Source: CAD feature listing. Evaluate the final solid. Frame: model axes, mm. A direction names the side the tool comes from. Coordinates: 2 decimals unless noted, no trailing zeros. Loops run counter-clockwise (first coordinate to the right, second up) from the corner with the lowest first, then second, coordinate; pieces in that order, holes last.
Item 1: Section query C-C, the plane y = 13. Return the cut outline in (x, z), then the cut area to 3 significant figures.
Item 2: Section query A-A, the plane x = 18. Return the cut outline in (y, z), then the cut area to 3 significant figures.
Item 3: Reachability of faces 1 (the flat face through (0, -26, 0)), 2 (the flat face through (-10.465, -7.697, 76.75)), 3 (the flat face through (-0.09, -47.92, 117.41)), 4 (the cylindrical face through (10.54, -18.81, 69)) from +Z, -Z, +X, -X, +Y, -Y: full face, straight path, thin tool, end or side. Return the list, or none.
Item 4: Pin query (flat end, axial travel): pin 1 Ø5 at (y, z) = (17, -5) entering from -X; pin 2 Ø10 at (x, y) = (-2.5, -21.5) entering from +Z; pin 3 Ø1.5 at (y, z) = (-12.5, 46.5) entering from -X; pin 4 Ø5 at (x, y) = (5.5, -40) entering from -Z. Return the tip coordinate at first contact, or that it passes through.
Item 5: Section query D-D, the plane x = -2. Return the cut outline in (y, z), then the cut area to 3 significant figures.
Item 6: Line query: probe 1 along Z at (x, y) = (-10, 18); probe 2 along X at (y, z) = (25.5, 15.5); probe 3 along Z at (x, y) = (-5.5, 0). Output: solid intervals per line, ascending.
Item 7: Section query B-B, the plane z = -12. Return the cut outline in (x, y).
```python
from build123d import *

# Parameters (mm, degrees)
BOSS_EXTRUDE2_DEPTH = 13
SKETCH1_4_R         = 35
BOSS_EXTRUDE3_DEPTH = 20
BOSS_EXTRUDE4_DEPTH = 8
SKETCH2_R           = 22
BOSS_EXTRUDE5_DEPTH = 12.5
CUT_EXTRUDE1_DEPTH  = 12.5


with BuildPart() as part:
    # Sketch1 → Boss-Extrude2 (new, symmetric)
    with BuildSketch(Plane(origin=(0, 0, 0), x_dir=(0, 0, -1), z_dir=(1, 0, 0))):
        with BuildLine():
            ThreePointArc((0, 35), (-32.769963209, 31.299429366), (-61.665057093, 15.404830876))
            Line((-61.665057093, 15.404830876), (-134.181781084, -45.443925478))
            Line((-134.181781084, -45.443925478), (-118.112090842, -64.595036556))
            Line((-118.112090842, -64.595036556), (-79.531665184, -32.222215616))
            ThreePointArc((-79.531665184, -32.222215616), (-50.616442429, -20.628497988), (-20.449595974, -28.40447191))
            ThreePointArc((-20.449595974, -28.40447191), (-33.310332608, 10.743451102), (0, 35))
        make_face()
        with BuildLine():
            Line((-107.958660037, -33.883372594), (-44.65586319, 19.233980892))
            ThreePointArc((-44.65586319, 19.233980892), (-43.34571286, 19.832159244), (-41.9077315, 19.751407541))
            ThreePointArc((-41.9077315, 19.751407541), (-40.085906415, 18.184292753), (-39.998801846, 15.782770696))
            ThreePointArc((-39.998801846, 15.782770696), (-42.92008559, 2.620353591), (-41.621711579, -10.799681718))
            ThreePointArc((-41.621711579, -10.799681718), (-42.152723603, -13.388818271), (-44.52547273, -14.553147883))
            ThreePointArc((-44.52547273, -14.553147883), (-69.329263161, -18.927231696), (-91.141343442, -31.520634046))
            Line((-91.141343442, -31.520634046), (-102.17357155, -40.777772582))
            ThreePointArc((-102.17357155, -40.777772582), (-104.363401607, -41.468223347), (-106.400067708, -40.408002082))
            Line((-106.400067708, -40.408002082), (-108.328430537, -38.109868752))
            ThreePointArc((-108.328430537, -38.109868752), (-109.018881302, -35.920038695), (-107.958660037, -33.883372594))
        make_face(mode=Mode.SUBTRACT)
    extrude(amount=BOSS_EXTRUDE2_DEPTH, both=True)

    # Sketch1_4 → Boss-Extrude3 (add, symmetric)
    with BuildSketch(Plane(origin=(0, 0, 0), x_dir=(0, 0, -1), z_dir=(1, 0, 0))):
        Circle(SKETCH1_4_R)
        with BuildLine():
            Line((22.550897352, -14.060833141), (16.517461106, -11.864841937))
            ThreePointArc((16.517461106, -11.864841937), (11.664928714, -16.659244691), (5.5, -19.579351255))
            Line((5.5, -19.579351255), (5.5, -26))
            Line((5.5, -26), (-5.5, -26))
            Line((-5.5, -26), (-5.5, -19.579351255))
            ThreePointArc((-5.5, -19.579351255), (-11.664928714, 16.659244691), (20.279682682, -1.528223108))
            Line((20.279682682, -1.528223108), (26.313118929, -3.724214312))
            Line((26.313118929, -3.724214312), (22.550897352, -14.060833141))
        make_face(mode=Mode.SUBTRACT)
    extrude(amount=BOSS_EXTRUDE3_DEPTH, both=True)

    # Sketch1_5 → Boss-Extrude4 (add, symmetric)
    with BuildSketch(Plane(origin=(0, 0, 0), x_dir=(0, 0, -1), z_dir=(1, 0, 0))):
        with BuildLine():
            Line((-108.328430537, -38.109868752), (-106.400067708, -40.408002082))
            ThreePointArc((-106.400067708, -40.408002082), (-104.363401607, -41.468223347), (-102.17357155, -40.777772582))
            Line((-102.17357155, -40.777772582), (-91.141343442, -31.520634046))
            ThreePointArc((-91.141343442, -31.520634046), (-69.329263161, -18.927231696), (-44.52547273, -14.553147883))
            ThreePointArc((-44.52547273, -14.553147883), (-42.152723603, -13.388818271), (-41.621711579, -10.799681718))
            ThreePointArc((-41.621711579, -10.799681718), (-42.92008559, 2.620353591), (-39.998801846, 15.782770696))
            ThreePointArc((-39.998801846, 15.782770696), (-40.085906415, 18.184292753), (-41.9077315, 19.751407541))
            ThreePointArc((-41.9077315, 19.751407541), (-43.34571286, 19.832159244), (-44.65586319, 19.233980892))
            Line((-44.65586319, 19.233980892), (-107.958660037, -33.883372594))
            ThreePointArc((-107.958660037, -33.883372594), (-109.018881302, -35.920038695), (-108.328430537, -38.109868752))
        make_face()
    extrude(amount=BOSS_EXTRUDE4_DEPTH, both=True)

    # Sketch2 → Boss-Extrude5 (add, symmetric)
    with BuildSketch(Plane(origin=(0, 29.828483461, 25.029069471), x_dir=(-1, 0, 0), z_dir=(0, -0.7660444431189768, -0.6427876096865408))):
        with Locations((0, -132)):
            Circle(SKETCH2_R)
        Polygon((6.5, -120.741669751), (-6.5, -120.741669751), (-13, -132), (-6.5, -143.258330249), (6.5, -143.258330249), (13, -132), align=None, mode=Mode.SUBTRACT)
    extrude(amount=BOSS_EXTRUDE5_DEPTH, both=True)

    # Sketch2_2 → Cut-Extrude1 (cut, symmetric)
    with BuildSketch(Plane(origin=(0, 29.828483461, 25.029069471), x_dir=(-1, 0, 0), z_dir=(0, -0.7660444431189768, -0.6427876096865408))):
        Polygon((6.5, -143.258330249), (13, -132), (6.5, -120.741669751), (-6.5, -120.741669751), (-13, -132), (-6.5, -143.258330249), align=None)
    extrude(amount=CUT_EXTRUDE1_DEPTH, both=True, mode=Mode.SUBTRACT)


solid = part.part
```
Verdict:
1. outline: (-20, -32.5) - (20, -32.5) - (20, -15.64) - (-20, -15.64) - close; (-20, 15.64) - (20, 15.64) - (20, 32.5) - (13, 32.5) - (13, 40.99) - (8, 40.99) - (8, 52.09) - (13, 52.09) - (13, 64.53) - (-13, 64.53) - (-13, 52.09) - (-8, 52.09) - (-8, 40.99) - (-13, 40.99) - (-13, 32.5) - (-20, 32.5) - close
1. area: 2,070 mm2
2. outline: (-72.73, 127.8) - (-56.46, 108.42) - (-37.31, 124.49) - (-53.57, 143.87) - close; circle Ø70 at (0, 0); hole (-26, -5.5) - (-19.58, -5.5) arc R20.34 ccw to (-11.86, -16.52) - (-14.06, -22.55) - (-3.72, -26.31) - (-1.53, -20.28) arc R20.34 ccw (long way) to (-19.58, 5.5) - (-26, 5.5) - close
2. area: 3,050 mm2
3. face 1: +X, -X
3. face 2: -X
3. face 3: -Y
3. face 4: +X
4. pin 1: passes through
4. pin 2: stops at z = 111.61
4. pin 3: stops at x = -8
4. pin 4: stops at z = 85.82
5. outline: (-78.68, 134.9) - (-71.83, 126.74) - (-52.68, 142.81) - (-59.53, 150.96) - close; (-57.36, 109.49) - (-32.22, 79.53) arc R50 cw to (-28.4, 20.45) arc R35 ccw (long way) to (35, 0) arc R85 ccw to (15.4, 61.67) - (-38.21, 125.56) - close; hole (-26, -5.5) - (-19.58, -5.5) arc R20.34 ccw to (-11.86, -16.52) - (-14.06, -22.55) - (-3.72, -26.31) - (-1.53, -20.28) arc R20.34 ccw (long way) to (-19.58, 5.5) - (-26, 5.5) - close
5. area: 6,050 mm2
6. probe 1: z = -30.02 to -9.47, 9.47 to 40, 46.13 to 58.41
6. probe 2: x = -20 to 20
6. probe 3: z = -35 to -20.34, 20.34 to 80.02
7. outline: (-20, -32.88) - (20, -32.88) - (20, -16.42) - (-20, -16.42) - close; (-20, 16.42) - (20, 16.42) - (20, 32.88) - (-20, 32.88) - close
